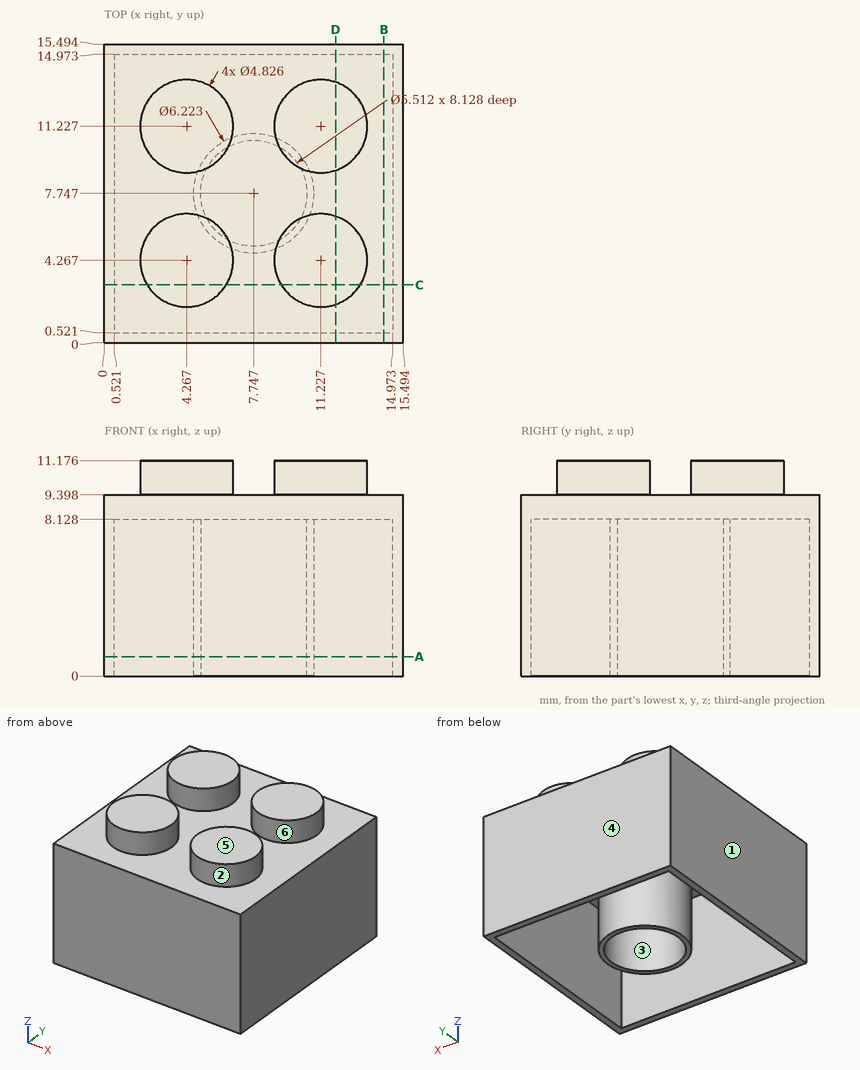
Source: three-view drawing plus pictorial views. Frame: mm from the lowest corner of the part. A direction names the side the tool comes from. Coordinates: 2 decimals unless noted, no trailing zeros. Order: outer loops, then holes, each group sorted by start corner. A loop starts at its lowest first (then second) coordinate and runs counter-clockwise, first axis right, second up.
1) Section C-C (y = 3). Return loops of the section in (x, z).
Result sheet:
outline: (0, 0) - (0.52, 0) - (0.52, 8.13) - (14.97, 8.13) - (14.97, 0) - (15.49, 0) - (15.49, 9.4) - (13.28, 9.4) - (13.28, 11.18) - (9.17, 11.18) - (9.17, 9.4) - (6.32, 9.4) - (6.32, 11.18) - (2.21, 11.18) - (2.21, 9.4) - (0, 9.4) - close
2) Section A-A (z = 1). Return loops of the section in (x, y).
Result sheet:
outline: (0, 0) - (15.49, 0) - (15.49, 15.49) - (0, 15.49) - close; circle Ø6.22 at (7.75, 7.75); hole (0.52, 0.52) - (14.97, 0.52) - (14.97, 14.97) - (0.52, 14.97) - close; hole circle Ø5.51 at (7.75, 7.75)
3) Set-up query: the marked faces 1, 2 and 3. Return all of +Z, -Z, +X, -X, +Y, -Y with unobstructed straight access to the full face (end or side cutting, diameter ignored); none if empty.
Result sheet:
face 1: +Z, -Z, -X, +Y, -Y
face 2: +Z
face 3: -Z
4) Draft query along Y for the marked faces 4, 5 and 6. Return one class per face: released by +Y, released by -Y, zero draft, split by the parting line, or undercut.
Result sheet:
face 4: released by +Y
face 5: zero draft
face 6: undercut
5) Ray query, probe 1 along X at (y, z) = (3, 2.75); probe 2 along Y at (x, z) = (5.25, 4) (1 decimal); probe 3 along Y at (x, z) = (8, 3.25). Return the intervals inside material, ascending.
Result sheet:
probe 1: x = 0 to 0.52, 14.97 to 15.49
probe 2: y = 0 to 0.5, 5.9 to 6.6, 8.9 to 9.6, 15 to 15.5
probe 3: y = 0 to 0.52, 4.65 to 5, 10.49 to 10.85, 14.97 to 15.49
6) First-contact query: P1, Ø4.5, axis at x = 6, y = 5.5, coming from the -Z side; P2, Ø1.5, axis at x = 11.5, y = 12.5, coming from the -Z side. Flat tips, straight axial feed; report the tip coordinate or a pass-through.
Result sheet:
P1: stops at z = 0
P2: stops at z = 8.13
7) Section B-B (x = 14.5). Return loops of the section in (y, z).
Result sheet:
outline: (0, 0) - (0.52, 0) - (0.52, 8.13) - (14.97, 8.13) - (14.97, 0) - (15.49, 0) - (15.49, 9.4) - (0, 9.4) - close
8) Section D-D (x = 12). Return loops of the section in (y, z).
Result sheet:
outline: (0, 0) - (0.52, 0) - (0.52, 8.13) - (14.97, 8.13) - (14.97, 0) - (15.49, 0) - (15.49, 9.4) - (13.51, 9.4) - (13.51, 11.18) - (8.94, 11.18) - (8.94, 9.4) - (6.55, 9.4) - (6.55, 11.18) - (1.98, 11.18) - (1.98, 9.4) - (0, 9.4) - close
